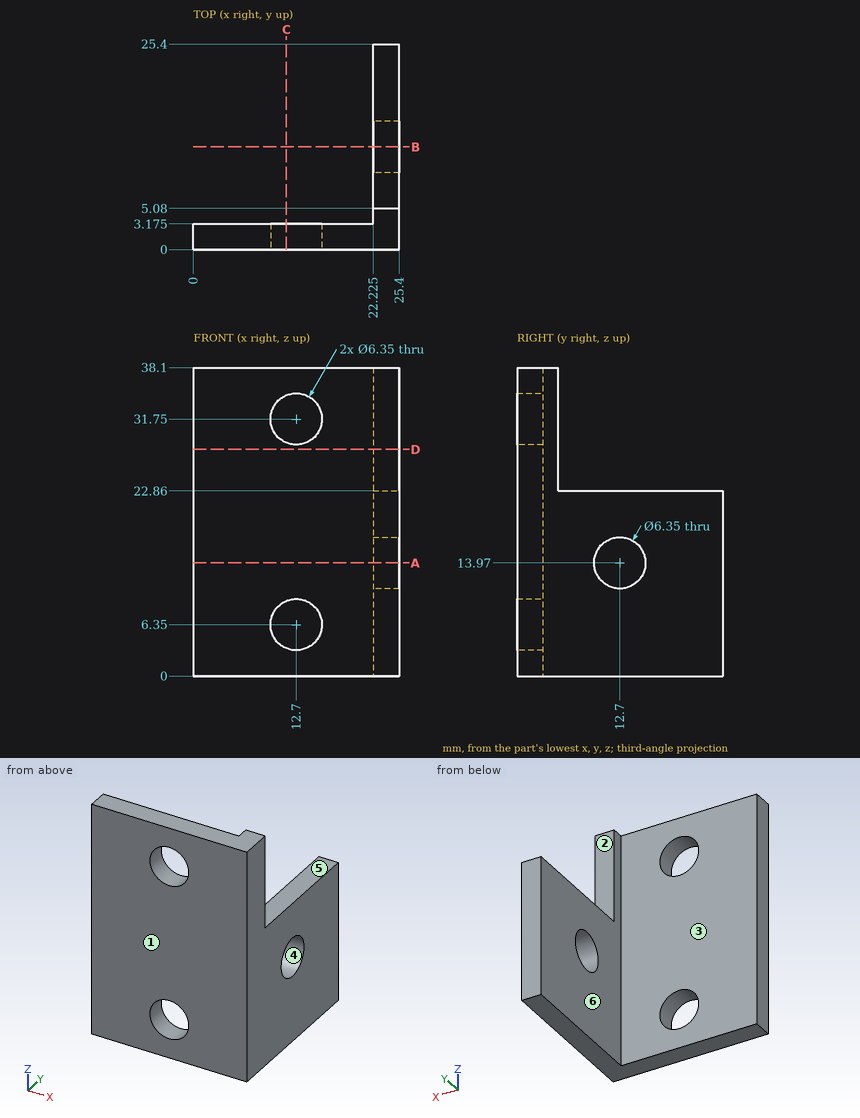
Can you work these out from the drawing? Everything is in mm from the part's minimum corner. A direction names the side the tool comes from. Coordinates: 2 decimals unless noted, no trailing zeros. Loops run counter-clockwise (first coordinate to the right, second up) from the corner with the lowest first, then second, coordinate; pieces in that order, holes last.
1. Imagine slicing it at B-B, the plane y = 12.7. Please give me the cut outline in (x, z) (3 decimals).
2. For P1, Ø3.5, axis at x = 23.5, y = 16, coming from the +Z side; P2, Ø10, axis at y = 12.7, z = 13.97, coming from the -X side (3 decimals); P3, Ø1.6, axis at x = 24, z = 27.5, coming from the +Y side, each with a flat end and sliding along its axis, tell me the tip position at first contact or that it passes through.
3. I need wall thicknesses on L1, parallel to X at y = 0.8, z = 31.75 (3 decimals); L2, parallel to Z at x = 15.5, y = 2.75; L3, parallel to Y at x = 7.75, z = 3 (3 decimals). Which ranges of each line are inside material? Lowest first, please.
4. For the marked faces 1, 2 and 3, which set-ups out of +Z, -Z, +X, -X, +Y, -Y let a thin tool reach every point of the face, with its end or its side?
5. Imagine slicing it at C-C, the plane x = 11.5. Please give me the cut outline in (y, z) (1 decimal).
6. Imagine slicing it at D-D, the plane z = 28. Please give me the cut outline in (x, y) (3 decimals), and give its area (3 significant figures).
7. If we mould it in two halves opening along Z, with no side actions, what happens to the marked faces 4, 5 and 6? For each: pulls with the +Z half, pulls with the -Z half, needs draft (parallel to the pull), parting line crosses it, or undercut.
8. Imagine slicing it at A-A, the plane z = 13.97. Please give me the cut outline in (x, y) (3 decimals).
Taken from the geometry:
1. outline: (22.225, 0) - (25.4, 0) - (25.4, 10.795) - (22.225, 10.795) - close; (22.225, 17.145) - (25.4, 17.145) - (25.4, 22.86) - (22.225, 22.86) - close
2. P1: stops at z = 22.86
2. P2: stops at x = 22.225
2. P3: stops at y = 5.08
3. L1: x = 0 to 9.525, 15.875 to 25.4
3. L2: z = 0 to 4.85, 7.85 to 30.25, 33.25 to 38.1
3. L3: y = 0 to 3.175
4. face 1: +Z, -Z, +X, -X, -Y
4. face 2: +Z, +X, -X, +Y
4. face 3: +Z, -Z, -X, +Y
5. outline: (0, 0) - (3.2, 0) - (3.2, 3.4) - (0, 3.4) - close; (0, 9.3) - (3.2, 9.3) - (3.2, 28.8) - (0, 28.8) - close; (0, 34.7) - (3.2, 34.7) - (3.2, 38.1) - (0, 38.1) - close
6. outline: (0, 0) - (25.4, 0) - (25.4, 5.08) - (22.225, 5.08) - (22.225, 3.175) - (0, 3.175) - close
6. area: 86.7 mm2
7. face 4: undercut
7. face 5: pulls with the +Z half
7. face 6: needs draft
8. outline: (0, 0) - (25.4, 0) - (25.4, 9.525) - (22.225, 9.525) - (22.225, 3.175) - (0, 3.175) - close; (22.225, 15.875) - (25.4, 15.875) - (25.4, 25.4) - (22.225, 25.4) - close
